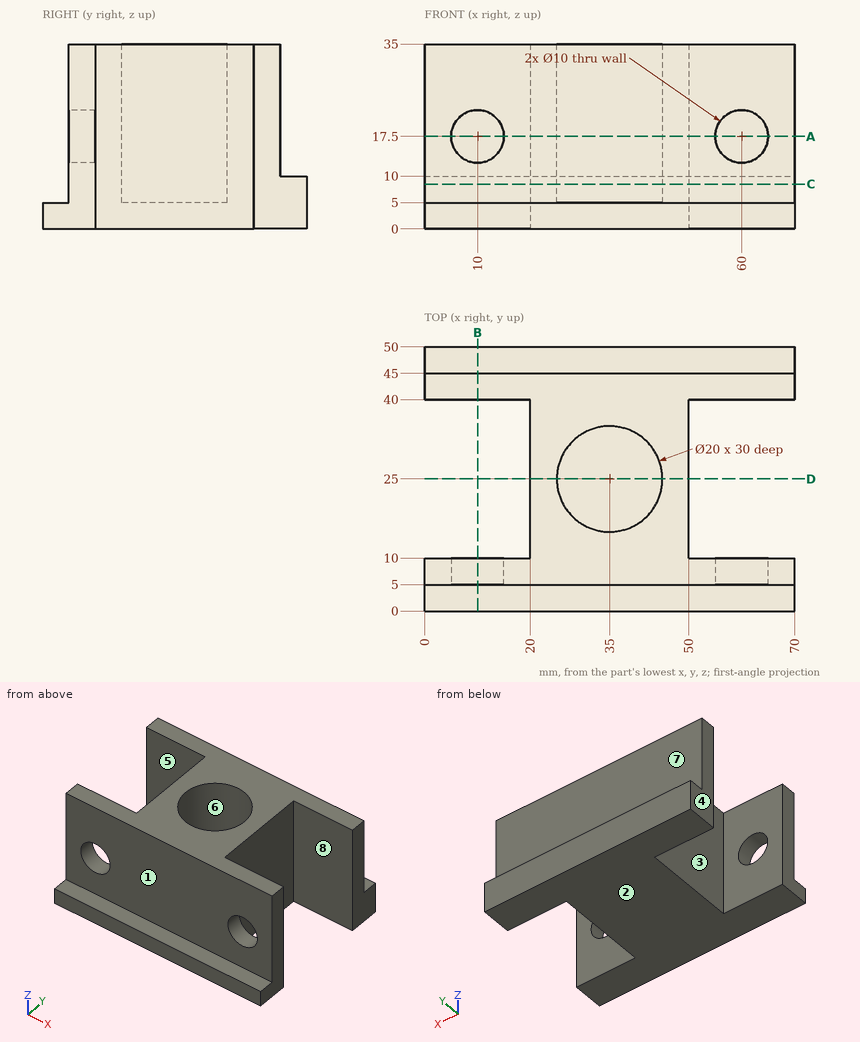
Verification items for this drawing (mm, ordinates from the low corner). A direction names the side the tool comes from. Round coordinates to 2 decimals unless told otherwise and drop trailing zeros. Order: outer loops, then holes, each group sorted by start corner. A loop starts at its lowest first (then second) coordinate and runs counter-clockwise, first axis right, second up.
1) Material ranges on line 1 (Y direction, x = 35, z = 16.5); line 2 (Z direction, x = 10, y = 6.45); line 3 (Y direction, x = 18, z = 28), recorded low to high.
Geometry says:
line 1: y = 5 to 15, 35 to 45
line 2: z = 0 to 12.5, 22.5 to 35
line 3: y = 5 to 10, 40 to 45
2) Cross-section at C-C, the plane z = 8.5. Record the cut outline in (x, y).
Geometry says:
outline: (0, 5) - (70, 5) - (70, 10) - (50, 10) - (50, 40) - (70, 40) - (70, 50) - (0, 50) - (0, 40) - (20, 40) - (20, 10) - (0, 10) - close; hole circle Ø20 at (35, 25)
3) Cross-section at A-A, the plane z = 17.5. Record the cut outline in (x, y).
Geometry says:
outline: (0, 5) - (5, 5) - (5, 10) - (0, 10) - close; (0, 40) - (20, 40) - (20, 10) - (15, 10) - (15, 5) - (55, 5) - (55, 10) - (50, 10) - (50, 40) - (70, 40) - (70, 45) - (0, 45) - close; (65, 5) - (70, 5) - (70, 10) - (65, 10) - close; hole circle Ø20 at (35, 25)
4) Depth check by flat-ended pin: pin 1 (9 mm diameter, centred on x = 51.5, z = 15, fed in from -Y); pin 2 (10 mm diameter, centred on x = 35, y = 29.5, fed in from +Z); pin 3 (2 mm diameter, centred on y = 42, z = 8, fed in from -X); pin 4 (6 mm diameter, centred on x = 10, z = 17.5, fed in from +Y). Enter the tip coordinate at first touch or a pass-through.
Geometry says:
pin 1: stops at y = 5
pin 2: stops at z = 5
pin 3: stops at x = 0
pin 4: stops at y = 45
5) Tool access check on the marked faces 4, 5, 6, 7 and 8. Record the directions out of +Z, -Z, +X, -X, +Y, -Y that give a thin tool (end or side, any length) a straight path to the whole face; none if there is none.
Geometry says:
face 4: +Z, -Z, -X, +Y, -Y
face 5: +Z, -Z, -X
face 6: +Z
face 7: +Z, +X, -X, +Y
face 8: +Z, -Z, +X
6) Cross-section at D-D, the plane y = 25. Record the cut outline in (x, z).
Geometry says:
outline: (20, 0) - (50, 0) - (50, 35) - (45, 35) - (45, 5) - (25, 5) - (25, 35) - (20, 35) - close
7) Draft check along Y on the marked faces 1, 2 and 3. Enter one of: +Y half, -Y half, draft (parallel to the pull), parting line (faces both ways), or undercut.
Geometry says:
face 1: -Y half
face 2: draft
face 3: undercut
8) Cross-section at B-B, the plane x = 10. Record the cut outline in (y, z), plus the area to 3 significant figures.
Geometry says:
outline: (0, 0) - (10, 0) - (10, 12.5) - (5, 12.5) - (5, 5) - (0, 5) - close; (5, 22.5) - (10, 22.5) - (10, 35) - (5, 35) - close; (40, 0) - (50, 0) - (50, 10) - (45, 10) - (45, 35) - (40, 35) - close
area: 375 mm2
